Source: three-view drawing plus pictorial views. Frame: mm from the lowest corner of the part. Coordinates: 2 decimals unless noted, no trailing zeros. Write each loop counter-clockwise with the first axis right and the second up, starting at its lowest first coordinate (ties: lowest second). Pieces come first, ordered by that corner, then holes. Notation, with made-up numbers: (16.5, 40.25) -> (68.5, 40.25) arc R18 ccw to (68.5, 46.25) -> close; hole circle Ø11 at (3.5, -12.75). An arc over 180 degrees is marked (long way). Write item = value, one per line.
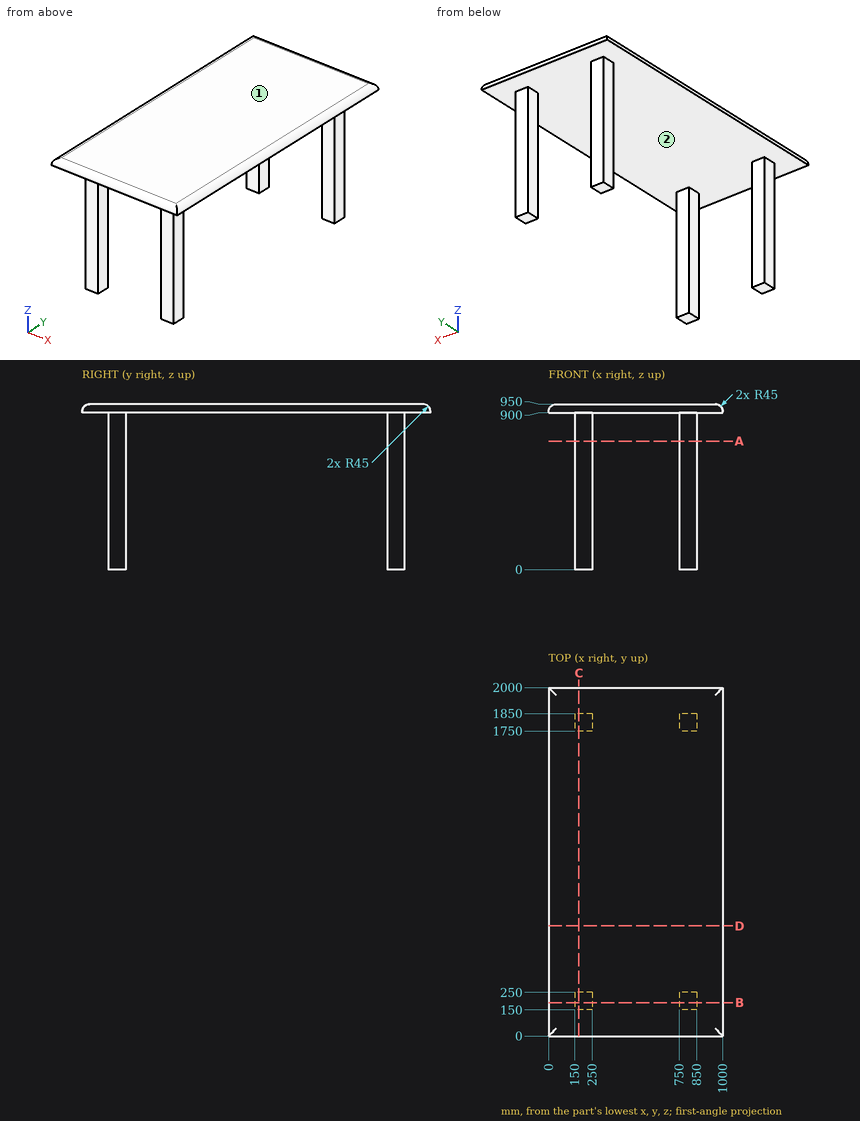
1) Cut plane D-D, the plane y = 632.5. Output: boundary loops of the cut face in (x, z).
Answer block:
outline = (0, 900) -> (1000, 900) -> (1000, 905) arc R45 ccw to (955, 950) -> (45, 950) arc R45 ccw to (0, 905) -> close
2) Material intervals for probe 1 along X at (y, z) = (163, 117.5); probe 2 along Y at (x, z) = (176.5, 769.5); probe 3 along Z at (x, y) = (718, 466.5), sorted ascending. Write a range as [from, to].
Answer block:
probe_1 = [150, 250], [750, 850]
probe_2 = [150, 250], [1750, 1850]
probe_3 = [900, 950]
3) First-contact query: pin 1 Ø8 at (x, z) = (770, 549.5) entering from +Y; pin 2 Ø6 at (x, z) = (251.5, 806.5) entering from -Y. Flat tips, straight axial feed; report the tip coordinate or a pass-through.
Answer block:
pin_1 = 1850
pin_2 = 150
4) Cut plane B-B, the plane y = 191.5. Output: boundary loops of the cut face in (x, z).
Answer block:
outline = (0, 900) -> (150, 900) -> (150, 0) -> (250, 0) -> (250, 900) -> (750, 900) -> (750, 0) -> (850, 0) -> (850, 900) -> (1000, 900) -> (1000, 905) arc R45 ccw to (955, 950) -> (45, 950) arc R45 ccw to (0, 905) -> close
5) Cut plane A-A, the plane z = 737. Output: boundary loops of the cut face in (x, y), and give its area (3 significant figures).
Answer block:
outline = (150, 150) -> (250, 150) -> (250, 250) -> (150, 250) -> close; (150, 1750) -> (250, 1750) -> (250, 1850) -> (150, 1850) -> close; (750, 150) -> (850, 150) -> (850, 250) -> (750, 250) -> close; (750, 1750) -> (850, 1750) -> (850, 1850) -> (750, 1850) -> close
area = 40,000 mm2
6) Pull-direction query (Y, two-part tool) for the marked faces 1 and 2; classes: +Y half, -Y half, draft (parallel to the pull), parting line (faces both ways), or undercut.
Answer block:
face_1 = draft
face_2 = undercut
7) Cut plane C-C, the plane x = 173. Output: boundary loops of the cut face in (y, z).
Answer block:
outline = (0, 900) -> (150, 900) -> (150, 0) -> (250, 0) -> (250, 900) -> (1750, 900) -> (1750, 0) -> (1850, 0) -> (1850, 900) -> (2000, 900) -> (2000, 905) arc R45 ccw to (1955, 950) -> (45, 950) arc R45 ccw to (0, 905) -> close
